Job drawing, mm, ordinate dimensions from the low corner. One solid piece. Coordinates: 2 decimals unless noted, no trailing zeros. Loops run counter-clockwise (first coordinate to the right, second up) from the corner with the lowest first, then second, coordinate; pieces in that order, holes last. Notation, with made-up numbers: M 14,2.5 L 28,2.5 A27 ccw 28,26.5 Z; hole C 38,86.5 d2. An arc over 180 degrees is marked long. Write each question's results on one line, items separated by ' | '. Start each with the question number.
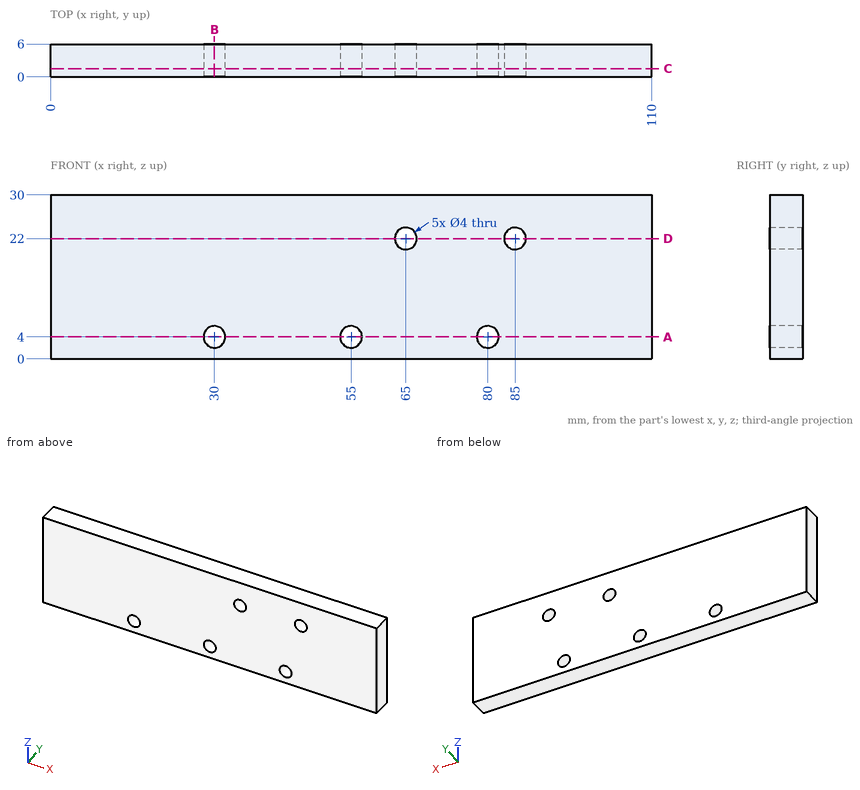
1. Wall check: line 1 along Z through (x, y) = (80, 4.3); line 2 along X through (y, z) = (3.5, 20.5); line 3 along X through (y, z) = (1.4, 2.75). Give the ranges that are in metal, low to high.
2. Band-saw the part on D-D, the plane z = 22. List the corners of the cut face in (x, y).
3. Band-saw the part on A-A, the plane z = 4. List the corners of the cut face in (x, y), plus the area to 3 significant figures.
4. Band-saw the part on C-C, the plane y = 1.5. List the corners of the cut face in (x, z).
5. Band-saw the part on B-B, the plane x = 30. List the corners of the cut face in (y, z).
Checked values:
1) line 1: 0 to 2, 6 to 30 | line 2: 0 to 63.68, 66.32 to 83.68, 86.32 to 110 | line 3: 0 to 28.44, 31.56 to 53.44, 56.56 to 78.44, 81.56 to 110
2) outline: M 0,0 L 63,0 L 63,6 L 0,6 Z; M 67,0 L 83,0 L 83,6 L 67,6 Z; M 87,0 L 110,0 L 110,6 L 87,6 Z
3) outline: M 0,0 L 28,0 L 28,6 L 0,6 Z; M 32,0 L 53,0 L 53,6 L 32,6 Z; M 57,0 L 78,0 L 78,6 L 57,6 Z; M 82,0 L 110,0 L 110,6 L 82,6 Z | area: 588 mm²
4) outline: M 0,0 L 110,0 L 110,30 L 0,30 Z; hole C 30,4 d4; hole C 55,4 d4; hole C 65,22 d4; hole C 80,4 d4; hole C 85,22 d4
5) outline: M 0,0 L 6,0 L 6,2 L 0,2 Z; M 0,6 L 6,6 L 6,30 L 0,30 Z
